Geometry: final body of the model. Coordinates: model frame, mm. A direction names the side the tool comes from. Give positions to 0.01 mm unless a question says otherwise; leave off trailing zeros. Loops run counter-clockwise (first coordinate to the right, second up) from the corner with the lowest first, then second, coordinate; pieces in that order, holes last.
1. Draft query along Y for faces 1 (the face through (-4, -2.54, -13)), 2 (the face through (-0.16, 28.936, -18.428)), 3 (the face through (0.16, 12.107, -12.911)), 4 (the face through (0, 40, -63.5)). Return one class per face: +Y half, -Y half, draft (parallel to the pull), parting line (faces both ways), or undercut.
2. Material intervals for line 1 along Y through (x, z) = (-2.5, -41); line 2 along Y through (x, z) = (-6, -14.5); line 3 along Y through (x, z) = (-2.5, -13.5), sorted ascending.
3. Access query for faces 5 (the face through (0, 2, -25.4)), 6 (the face through (-1.77, -1.25, -12.52)), 7 (the face through (0, -3, 0)), 8 (the face through (0.16, 23.106, -33.285)). Directions: +Z, -Z, +X, -X, +Y, -Y. A direction counts if a zero-diameter tool reaches every point of the face in a straight line with its end or side. Return the directions, or none.
4. Section D-D, the plane x = 9.25. Output: boundary loops of the cut face in (y, z), then the cut area to 3 significant figures.
5. Section B-B, the plane y = 8.5. Output: boundary loops of the cut face in (x, z).
6. Section A-A, the plane x = -4.25. Output: boundary loops of the cut face in (y, z), then the cut area to 3 significant figures.
7. Section C-C, the plane z = -49. Output: boundary loops of the cut face in (x, y).
8. First-contact query: P1, Ø2, axis at x = 2, y = 6.5, coming from the +Z side; P2, Ø4.5, axis at x = 2.5, y = -2.5, coming from the +Z side; P3, Ø0.8, axis at y = -3, z = -15.5, coming from the -X side. Flat tips, straight axial feed; report the tip coordinate or a pass-through.
from build123d import *

# Parameters (mm, degrees)
F1_DEPTH = 5.08
F2_DEPTH = 2.54
F4_DEPTH = 1.524
F6_DEPTH = 22.86
F8_DEPTH = 25.4


with BuildPart() as f1:
    # F0 (on Front) → F1 (new body)
    with BuildSketch(Plane.XZ):
        Polygon((11.43, 25.4), (-11.43, 25.4), (-11.43, -25.4), (-6.35, -25.4), (-6.35, 0), (-1.27, 0), (1.27, 0), (6.35, 0), (6.35, -25.4), (11.43, -25.4), align=None)
        Polygon((-6.35, 0), (-6.35, -25.4), (-2.286, -25.4), (-1.27, 0), align=None)
        Polygon((-1.27, 0), (-2.286, -25.4), (2.032, -25.4), (1.27, 0), align=None)
        Polygon((2.032, -25.4), (6.35, -25.4), (6.35, 0), (1.27, 0), align=None)
    extrude(amount=-F1_DEPTH)

    # F0 (on Front) → F2 (join)
    with BuildSketch(Plane.XZ):
        Polygon((-1.27, 0), (-2.286, -25.4), (2.032, -25.4), (1.27, 0), align=None)
    extrude(amount=F2_DEPTH)

    # F3 (on face) → F4 (join)
    with BuildSketch(Plane.XZ.offset(2.54)):
        Polygon((6.313071, 0), (1.27, 0), (2.032, -25.4), (6.313071, -25.4), align=None)
        Polygon((1.27, 0), (-1.27, 0), (-2.286, -25.4), (2.032, -25.4), align=None)
        Polygon((-1.27, 0), (-6.567071, 0), (-6.567071, -25.4), (-2.286, -25.4), align=None)
    extrude(amount=F4_DEPTH)

    # F5 (on face) → F6 (join, through all)
    with BuildSketch(Plane(origin=(-11.43, 0, 0), x_dir=(0, -1, 0), z_dir=(-1, 0, 0))):
        Polygon((-5.08, -25.4), (-5.08, 25.4), (-53.4693, -63.5), (-25.275299, -63.5), align=None)
    extrude(amount=-F6_DEPTH)

    # F7 (on face) → F8 (cut)
    with BuildSketch(Plane.YZ.offset(11.43)):
        Polygon((18.372589, -2.824009), (4.645219, 22.132182), (6.014857, -22.718789), align=None)
        Polygon((7.461059, -25.4), (26.760479, -61.180491), (19.348416, -4.59805), align=None)
        Polygon((28.510716, -61.180491), (50.472081, -61.180491), (21.645763, -8.774598), align=None)
    extrude(amount=-F8_DEPTH, mode=Mode.SUBTRACT)


solid = f1.part
Answers below:
1. face 1: undercut
1. face 2: +Y half
1. face 3: undercut
1. face 4: draft
2. line 1: y = 13.35 to 15.88, 24.12 to 25.87, 39.37 to 41.22
2. line 2: y = -4.06 to -2.54, 0 to 5.76, 11.12 to 13.69, 20.65 to 22.4, 24.8 to 26.8
2. line 3: y = -4.06 to -2.54, 0 to 5.73, 11.74 to 14.26, 20.51 to 22.26, 24.25 to 26.25
3. face 5: -Z, +X, -X, -Y
3. face 6: +Z, -X
3. face 7: +Z, +X, -X, -Y
3. face 8: +X, -X
4. outline: (0, -25.4) - (5.08, -25.4) - (25.28, -63.5) - (53.47, -63.5) - (5.08, 25.4) - (0, 25.4) - close; hole (4.65, 22.13) - (6.01, -22.72) - (18.37, -2.82) - close; hole (7.46, -25.4) - (26.76, -61.18) - (19.35, -4.6) - close; hole (21.65, -8.77) - (28.51, -61.18) - (50.47, -61.18) - close
4. area: 745 mm2
5. outline: (-11.43, -31.85) - (11.43, -31.85) - (11.43, -27.33) - (-11.43, -27.33) - close; (-11.43, -23.58) - (11.43, -23.58) - (11.43, -18.72) - (-11.43, -18.72) - close; (-11.43, 15.12) - (11.43, 15.12) - (11.43, 19.12) - (-11.43, 19.12) - close
6. outline: (-4.06, -25.4) - (-2.54, -25.4) - (-2.54, 0) - (-4.06, 0) - close; (0, -25.4) - (5.08, -25.4) - (25.28, -63.5) - (53.47, -63.5) - (5.08, 25.4) - (0, 25.4) - close; hole (4.65, 22.13) - (6.01, -22.72) - (18.37, -2.82) - close; hole (7.46, -25.4) - (26.76, -61.18) - (19.35, -4.6) - close; hole (21.65, -8.77) - (28.51, -61.18) - (50.47, -61.18) - close
6. area: 783 mm2
7. outline: (-11.43, 17.59) - (11.43, 17.59) - (11.43, 20.19) - (-11.43, 20.19) - close; (-11.43, 25.16) - (11.43, 25.16) - (11.43, 26.92) - (-11.43, 26.92) - close; (-11.43, 43.77) - (11.43, 43.77) - (11.43, 45.58) - (-11.43, 45.58) - close
8. P1: stops at z = 24.63
8. P2: stops at z = 0
8. P3: stops at x = -6.57
